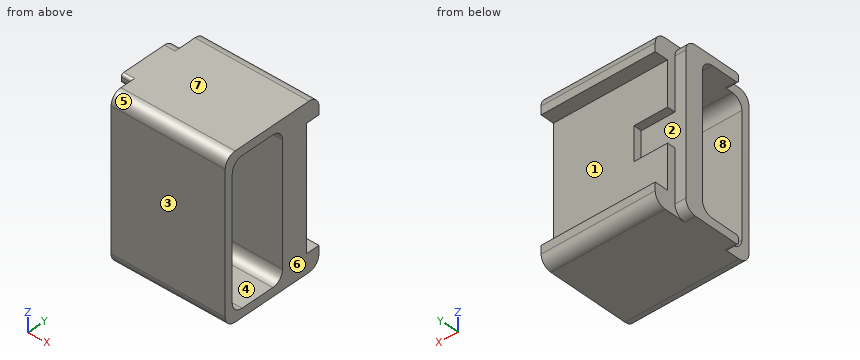
from build123d import *

# Parameters (mm, degrees)
BOSS_EXTRUDE1_DEPTH     = 21
SKETCH5_W               = 6.2
SKETCH5_H               = 6.2
CUT_EXTRUDE1_DEPTH      = 4
CUT_EXTRUDE2_DEPTH      = 28.364438602
CUT_EXTRUDE2_DEPTH_BACK = 28.364438602
SKETCH9_W               = 24.284850455
SKETCH9_H               = 22.464844075
CUT_EXTRUDE3_DEPTH      = 2.5
BOSS_EXTRUDE2_DEPTH     = 2


with BuildPart() as part:
    # Sketch3 → Boss-Extrude1 (new body)
    with BuildSketch(Plane(origin=(0, 0, 0), x_dir=(0, 0, -1), z_dir=(1, 0, 0))):
        with BuildLine():
            Line((-12.75, -9.5), (12.75, -9.5))
            ThreePointArc((12.75, -9.5), (14.164213562, -8.914213562), (14.75, -7.5))
            Line((14.75, -7.5), (14.75, 7.5))
            ThreePointArc((14.75, 7.5), (14.164213562, 8.914213562), (12.75, 9.5))
            Line((12.75, 9.5), (-12.75, 9.5))
            ThreePointArc((-12.75, 9.5), (-14.164213562, 8.914213562), (-14.75, 7.5))
            Line((-14.75, 7.5), (-14.75, -7.5))
            ThreePointArc((-14.75, -7.5), (-14.164213562, -8.914213562), (-12.75, -9.5))
        make_face()
    extrude(amount=BOSS_EXTRUDE1_DEPTH)

    # Sketch5 → Cut-Extrude1 (cut)
    with BuildSketch(Plane(origin=(0, 9.5, 0), x_dir=(1, 0, 0), z_dir=(0, 1, 0))):
        with Locations((3.1, 0)):
            Rectangle(SKETCH5_W, SKETCH5_H)
    extrude(amount=-CUT_EXTRUDE1_DEPTH, mode=Mode.SUBTRACT)

    # Sketch7 → Cut-Extrude2 (cut, two sides: drawn at the far end of the back side and taken through both)
    with BuildSketch(Plane.ZY.offset(-CUT_EXTRUDE2_DEPTH_BACK)):
        with BuildLine():
            Line((-11.147623693, -8.072928754), (11.147623693, -8.072928754))
            ThreePointArc((11.147623693, -8.072928754), (12.561837255, -7.487142316), (13.147623693, -6.072928754))
            Line((13.147623693, -6.072928754), (13.147623693, 0.135263404))
            ThreePointArc((13.147623693, 0.135263404), (12.561837255, 1.549476966), (11.147623693, 2.135263404))
            Line((11.147623693, 2.135263404), (-11.147623693, 2.135263404))
            ThreePointArc((-11.147623693, 2.135263404), (-12.561837255, 1.549476966), (-13.147623693, 0.135263404))
            Line((-13.147623693, 0.135263404), (-13.147623693, -6.072928754))
            ThreePointArc((-13.147623693, -6.072928754), (-12.561837255, -7.487142316), (-11.147623693, -8.072928754))
        make_face()
    extrude(amount=CUT_EXTRUDE2_DEPTH + CUT_EXTRUDE2_DEPTH_BACK, mode=Mode.SUBTRACT)

    # Sketch9 → Cut-Extrude3 (cut)
    with BuildSketch(Plane(origin=(0, 9.5, 0), x_dir=(1, 0, 0), z_dir=(0, 1, 0))):
        with Locations((12.142425228, 0.007615305)):
            Rectangle(SKETCH9_W, SKETCH9_H)
    extrude(amount=-CUT_EXTRUDE3_DEPTH, mode=Mode.SUBTRACT)

    # Sketch11 → Boss-Extrude2 (add)
    with BuildSketch(Plane.ZY):
        with BuildLine():
            Line((-13.647623693, -5.23512894), (-14.25, -5.23512894))
            ThreePointArc((-14.25, -5.23512894), (-14.603553391, -5.088682331), (-14.75, -4.73512894))
            Line((-14.75, -4.73512894), (-14.75, 3.5))
            ThreePointArc((-14.75, 3.5), (-14.164213562, 4.914213562), (-12.75, 5.5))
            Line((-12.75, 5.5), (12.75, 5.5))
            ThreePointArc((12.75, 5.5), (14.164213562, 4.914213562), (14.75, 3.5))
            Line((14.75, 3.5), (14.75, -4.73512894))
            ThreePointArc((14.75, -4.73512894), (14.603553391, -5.088682331), (14.25, -5.23512894))
            Line((14.25, -5.23512894), (13.647623693, -5.23512894))
            ThreePointArc((13.647623693, -5.23512894), (13.294070302, -5.088682331), (13.147623693, -4.73512894))
            Line((13.147623693, -4.73512894), (13.147623693, 0.135263404))
            ThreePointArc((13.147623693, 0.135263404), (12.561837255, 1.549476966), (11.147623693, 2.135263404))
            Line((11.147623693, 2.135263404), (-11.147623693, 2.135263404))
            ThreePointArc((-11.147623693, 2.135263404), (-12.561837255, 1.549476966), (-13.147623693, 0.135263404))
            Line((-13.147623693, 0.135263404), (-13.147623693, -4.73512894))
            ThreePointArc((-13.147623693, -4.73512894), (-13.294070302, -5.088682331), (-13.647623693, -5.23512894))
        make_face()
    extrude(amount=BOSS_EXTRUDE2_DEPTH)


solid = part.part
Input: part model. Units: mm. Frame: model coordinates. Face numbers are marked on the shaded views. A direction names the side the tool comes from. Coordinates: 2 decimals unless noted, no trailing zeros. Loops run counter-clockwise (first coordinate to the right, second up) from the corner with the lowest first, then second, coordinate; pieces in that order, holes last.
(1) Section A-A on z = 2. Return the cut outline in (x, y).
(2) Section C-C on x = 13.5. Return the cut outline in (y, z).
(3) Material intervals for probe 1 along Z at (x, y) = (0, -4.25); probe 2 along Y at (x, z) = (7.5, 11); probe 3 along X at (y, z) = (6, 9.5), sorted ascending.
(4) Pull-direction query (Z, two-part tool) for the marked faces 6, 7 and 8; classes: released by +Z, released by -Z, zero draft, split by the parting line, or undercut.
(5) First-contact query: pin 1 Ø5 at (y, z) = (-6.5, 1) entering from -X; pin 2 Ø1.6 at (y, z) = (6, 0.5) entering from -X; pin 3 Ø1.2 at (x, y) = (13, 8.5) entering from +Z; pin 4 Ø0.5 at (x, z) = (-0.5, -14) entering from -Y. Flat tips, straight axial feed; report the tip coordinate or a pass-through.
(6) Set-up query: the marked faces 1, 2, 3, 4 and 5. Return all of +Z, -Z, +X, -X, +Y, -Y with unobstructed straight access to the full face (end or side cutting, diameter ignored); none if empty.
(7) Section D-D on z = -5.5. Return the cut outline in (x, y), then the cut area to 3 significant figures.
(8) Section B-B on y = -0.5. Return the cut outline in (x, z).
Data:
1. outline: (-2, 2.14) - (21, 2.14) - (21, 7) - (6.2, 7) - (6.2, 5.5) - (-2, 5.5) - close; (0, -9.5) - (21, -9.5) - (21, -8.07) - (0, -8.07) - close
2. outline: (-9.5, -12.75) arc R2 ccw to (-7.5, -14.75) - (7.5, -14.75) arc R2 ccw to (9.5, -12.75) - (9.5, -11.24) - (7, -11.24) - (7, 11.22) - (9.5, 11.22) - (9.5, 12.75) arc R2 ccw to (7.5, 14.75) - (-7.5, 14.75) arc R2 ccw to (-9.5, 12.75) - close; hole (-8.07, -11.15) arc R2 ccw to (-6.07, -13.15) - (0.14, -13.15) arc R2 ccw to (2.14, -11.15) - (2.14, 11.15) arc R2 ccw to (0.14, 13.15) - (-6.07, 13.15) arc R2 ccw to (-8.07, 11.15) - close
3. probe 1: z = -14.75 to -13.15, 13.15 to 14.75
3. probe 2: y = -9.5 to -8.07, 2.14 to 7
3. probe 3: x = 0 to 21
4. face 6: zero draft
4. face 7: released by +Z
4. face 8: undercut
5. pin 1: stops at x = 0
5. pin 2: stops at x = -2
5. pin 3: stops at z = 14.71
5. pin 4: stops at y = -5.24
6. face 1: +X, -X, +Y
6. face 2: -X, +Y
6. face 3: +Z, -Z, +X, -X, -Y
6. face 4: +X, -X
6. face 5: +Z, +X, -X, -Y
7. outline: (-2, 2.14) - (21, 2.14) - (21, 7) - (0, 7) - (0, 5.5) - (-2, 5.5) - close; (0, -9.5) - (21, -9.5) - (21, -8.07) - (0, -8.07) - close
7. area: 139 mm2
8. outline: (-2, -14.75) - (21, -14.75) - (21, -13.15) - (-2, -13.15) - close; (-2, 13.15) - (21, 13.15) - (21, 14.75) - (-2, 14.75) - close
